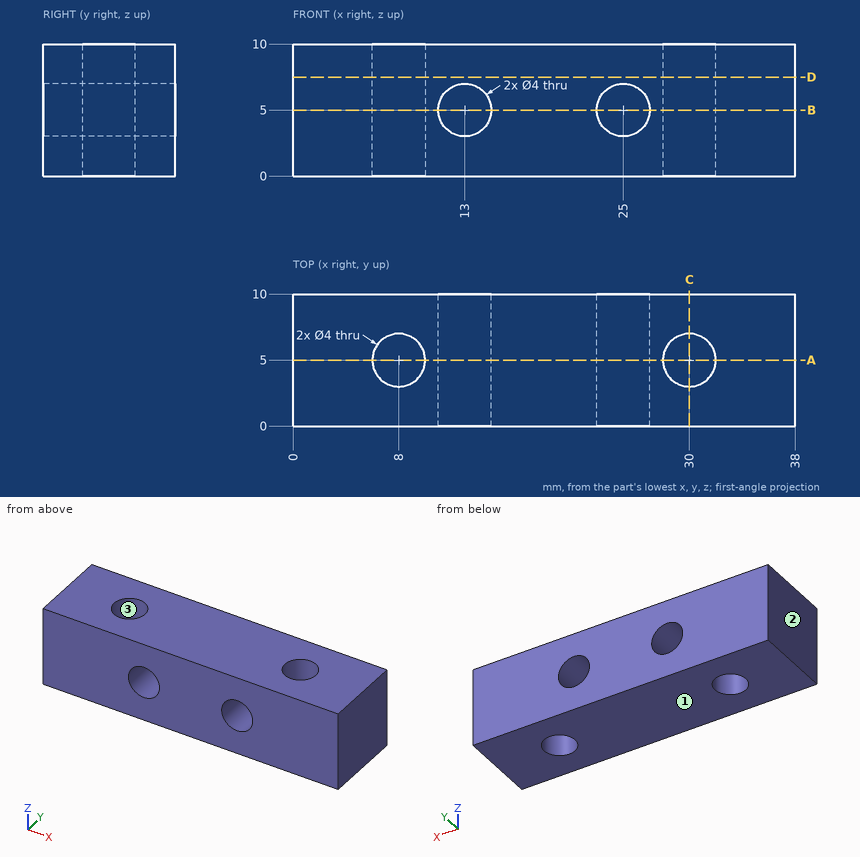
Source: three-view drawing plus pictorial views. Frame: mm from the lowest corner of the part. Round coordinates to 2 decimals unless told otherwise and drop trailing zeros. Loops run counter-clockwise (first coordinate to the right, second up) from the corner with the lowest first, then second, coordinate; pieces in that order, holes last.
1. Section query C-C on x = 30. Output: boundary loops of the cut face in (y, z).
2. Mould query, pull axis X, two halves, no side actions, for the marked faces 1, 2 and 3. Classes: released by +X, released by -X, zero draft, split by the parting line, or undercut.
3. Section query A-A on y = 5. Output: boundary loops of the cut face in (x, z), and give its area (3 significant figures).
4. Section query B-B on z = 5. Output: boundary loops of the cut face in (x, y).
5. Section query D-D on z = 7.5. Output: boundary loops of the cut face in (x, y).
6. Ray query, L1, parallel to X at y = 8, z = 5; L2, parallel to Y at x = 8, z = 6.5; L3, parallel to X at y = 4.25, z = 5. Return the intervals inside material, ascending.
Answers below:
1. outline: (0, 0) - (3, 0) - (3, 10) - (0, 10) - close; (7, 0) - (10, 0) - (10, 10) - (7, 10) - close
2. face 1: zero draft
2. face 2: released by -X
2. face 3: undercut
3. outline: (0, 0) - (6, 0) - (6, 10) - (0, 10) - close; (10, 0) - (28, 0) - (28, 10) - (10, 10) - close; (32, 0) - (38, 0) - (38, 10) - (32, 10) - close; hole circle Ø4 at (13, 5); hole circle Ø4 at (25, 5)
3. area: 275 mm2
4. outline: (0, 0) - (11, 0) - (11, 10) - (0, 10) - close; (15, 0) - (23, 0) - (23, 10) - (15, 10) - close; (27, 0) - (38, 0) - (38, 10) - (27, 10) - close; hole circle Ø4 at (8, 5); hole circle Ø4 at (30, 5)
5. outline: (0, 0) - (38, 0) - (38, 10) - (0, 10) - close; hole circle Ø4 at (8, 5); hole circle Ø4 at (30, 5)
6. L1: x = 0 to 11, 15 to 23, 27 to 38
6. L2: y = 0 to 3, 7 to 10
6. L3: x = 0 to 6.15, 9.85 to 11, 15 to 23, 27 to 28.15, 31.85 to 38
